from build123d import *

# Parameters (mm, degrees)
F0_R     = 10.35
F1_DEPTH = 56
F2_R     = 11.5
F3_DEPTH = 25
F5_DEPTH = 25
F6_R     = 4
F7_DEPTH = 25
F8_R     = 3.25
F9_DEPTH = 30
F10_SIZE = 3.25


with BuildPart() as f1:
    # F0 (on Front) → F1 (new body)
    with BuildSketch(Plane.XZ):
        Circle(F0_R)
    extrude(amount=F1_DEPTH)

    # F2 (on face) → F3 (join)
    with BuildSketch(Plane(origin=(0, 0, 0), x_dir=(-1, 0, 0), z_dir=(0, 1, 0))):
        Circle(F2_R)
    extrude(amount=F3_DEPTH)

    # F4 (on face) → F5 (cut, through all)
    with BuildSketch(Plane(origin=(0, 25, 0), x_dir=(-1, 0, 0), z_dir=(0, 1, 0))):
        with BuildLine():
            Line((-9.5, -6.4807406984), (-9.5, 6.4807406984))
            ThreePointArc((-9.5, 6.4807406984), (-11.5, 0), (-9.5, -6.4807406984))
        make_face()
        with BuildLine():
            ThreePointArc((11.5, 0), (10.9886304879, 3.3911649916), (9.5, 6.4807406984))
            Line((9.5, 6.4807406984), (9.5, -6.4807406984))
            ThreePointArc((9.5, -6.4807406984), (10.9886304879, -3.3911649916), (11.5, 0))
        make_face()
    extrude(amount=-F5_DEPTH, mode=Mode.SUBTRACT)

    # F6 (on face) → F7 (cut)
    with BuildSketch(Plane(origin=(-9.5, 0, 0), x_dir=(0, -1, 0), z_dir=(-1, 0, 0))):
        with Locations((-12.5, 0)):
            Circle(F6_R)
    extrude(amount=-F7_DEPTH, mode=Mode.SUBTRACT)

    # F8 (on face) → F9 (cut)
    with BuildSketch(Plane.XZ.offset(56)):
        Circle(F8_R)
    extrude(amount=-F9_DEPTH, mode=Mode.SUBTRACT)

    # F10
    f10_edges = [f1.edges().sort_by_distance(p)[0] for p in [
        (-3.25, -26, 0),
    ]]
    chamfer(f10_edges, length=F10_SIZE)


solid = f1.part
Check sheet for the modelled part. Datum: model origin and axes. Units: mm. A direction names the side the tool comes from. Give positions to 0.01 mm unless a question says otherwise; leave off trailing zeros. Loops run counter-clockwise (first coordinate to the right, second up) from the corner with the lowest first, then second, coordinate; pieces in that order, holes last. Notation, with made-up numbers: M 44,61 L 65,61 A34 ccw 65,92 Z; hole C 6.25,54 d6. An arc over 180 degrees is marked long. Answer as a JSON object with one key per item and string values. Group by question number.
Q1. Cross-section at B-B on x = -7. Record the cut outline in (y, z), then the cut area to 3 significant figures.
Q2. Go/stop test with flat-tipped pins: P1, Ø0.7, axis at x = -10, z = 0, coming from the +Y side; P2, Ø6, axis at x = 8, y = -1.5, coming from the +Z side; P3, Ø13, axis at y = 12.5, z = 0, coming from the +X side. Record where each tip stops, or that it passes through.
Q3. Release check for a two-part mould opening along Z. For faces 5 (the cylindrical face through (0.2, 12.3, -11.5)), 6 (the conical face through (0, -27, 1)), 7 (the flat face through (0, 0, 11)), 8 (the cylindrical face through (-0.1, 15.7, -2.4)) record: released by +Z, released by -Z, zero draft, split by the parting line, or undercut.
Q4. Cross-section at C-C on z = -9.25. Record the cut outline in (x, y), then the cut area to 3 significant figures.
Q5. Material ranges on line 1 along Z through (x, y) = (-0.5, 12.5); line 2 along Y through (x, z) = (-8, 2); line 3 along Z through (x, y) = (3, 9.5), recorded low to high. Write a range as [from, to].
Q6. Cross-section at D-D on x = 6. Record the cut outline in (y, z).
Q7. Cross-section at A-A on y = 12.5. Record the cut outline in (x, z).
Q8. Access from +Z, -Z, +X, -X, +Y, -Y to the whole of each face (thin tool, end or side, straight path). Record for faces 1 (the flat face through (-9.5, 15.5, 3)), 2 (the flat face through (0, 0, -11)), 3 (the flat face through (9.5, 15.5, -3)), 4 (the cylindrical face through (-8.21, -27.61, -6.3)).
Evaluation:
{
 "1": {"outline": "M -56,-7.62 L 0,-7.62 L 0,-9.12 L 25,-9.12 L 25,9.12 L 0,9.12 L 0,7.62 L -56,7.62 Z; hole C 12.5,0 d8", "area": "1,260 mm2"},
 "2": {"P1": "stops at y = 0", "P2": "stops at z = 10.15", "P3": "stops at x = 9.5"},
 "3": {"face 5": "released by -Z", "face 6": "undercut", "face 7": "zero draft", "face 8": "undercut"},
 "4": {"outline": "M -6.83,0 L -4.64,0 L -4.64,-56 L 4.64,-56 L 4.64,0 L 6.83,0 L 6.83,25 L -6.83,25 Z", "area": "862 mm2"},
 "5": {"line 1": "z = [-11.49, -4], [4, 11.49]", "line 2": "y = [-56, 9.04], [15.96, 25]", "line 3": "z = [-11.1, -2.65], [2.65, 11.1]"},
 "6": {"outline": "M -56,-8.43 L 0,-8.43 L 0,-9.81 L 25,-9.81 L 25,9.81 L 0,9.81 L 0,8.43 L -56,8.43 Z; hole C 12.5,0 d8"},
 "7": {"outline": "M -9.5,-6.48 A11.5 ccw 9.5,-6.48 L 9.5,-4 L -9.5,-4 Z; M -9.5,4 L 9.5,4 L 9.5,6.48 A11.5 ccw -9.5,6.48 Z"},
 "8": {"face 1": "+Z, -Z, -X, +Y", "face 2": "-Z, -Y", "face 3": "+Z, -Z, +X, +Y", "face 4": "-Y"}
}
